from build123d import *

# Parameters (mm, degrees)
SKETCH_1_R               = 139
EXTRUDE_1_DEPTH          = 10
CUT_EXTRUDE_578_DEPTH    = 8
PATTERN_CIRCULAR_1_COUNT = 14
SKETCH_3_R               = 51
CUT_EXTRUDE_927_DEPTH    = 197.829875781
SKETCH_5_R               = 10
CUT_EXTRUDE_1077_DEPTH   = 197.738404995
PATTERN_CIRCULAR_2_COUNT = 14
HOLE_WIZARD_M3_D         = 3.6
MIRROR_2_COPY_1_D        = 3.6
M5SUPPORTINGPOLE_D       = 5.8
M5_SUPPORTING_POLE_D     = 5.8
MIRROR_4_COPY_1_D        = 5.8
MIRROR_4_COPY_2_D        = 5.8
MIRROR_4_COPY_3_D        = 5.8
SKETCH_15_R              = 5.1
CUT_EXTRUDE_7_DEPTH      = 5
MIRROR_6_COPY_1_SKETCH_R = 5.1
MIRROR_6_COPY_1_DEPTH    = 5
SKETCH_16_R              = 60
SKETCH_16_R_2            = 51
CUT_EXTRUDE_8_DEPTH      = 8
SKETCH_18_R              = 2.5
CUT_EXTRUDE_10_DEPTH     = 197.829875781


with BuildPart() as part:
    # ｽｹｯﾁ1 → ﾎﾞｽ - 押し出し1 (new body)
    with BuildSketch(Plane(origin=(0, 0, 0), x_dir=(1, 0, 0), z_dir=(0, 1, 0))):
        with Locations(Location((0, 0, 0), (0, 0, 270))):
            Circle(SKETCH_1_R)
    extrude(amount=EXTRUDE_1_DEPTH)

    # ｽｹｯﾁ2 → Cut-Extrude 578 (cut)
    with BuildSketch(Plane.XZ):
        with BuildLine():
            Line((18.5, 119), (18.5, 85))
            ThreePointArc((18.5, 85), (0, 66.5), (-18.5, 85))
            Line((-18.5, 85), (-18.5, 119))
            ThreePointArc((-18.5, 119), (0, 137.5), (18.5, 119))
        make_face()
    cut_extrude_578 = extrude(amount=-CUT_EXTRUDE_578_DEPTH, mode=Mode.SUBTRACT)

    # 円形ﾊﾟﾀｰﾝ1: Cut-Extrude 578 ×14 about axis
    pattern_circular_1_axis = Axis((0, 0, 0), (0, 1, 0))
    for i in range(1, PATTERN_CIRCULAR_1_COUNT):
        add(cut_extrude_578.rotate(pattern_circular_1_axis, i * 360 / PATTERN_CIRCULAR_1_COUNT), mode=Mode.SUBTRACT)

    # ｽｹｯﾁ3 → Cut-Extrude 927 (cut, through all)
    with BuildSketch(Plane(origin=(0, 0, 0), x_dir=(-1, 0, 0), z_dir=(0, -1, 0))):
        with Locations(Location((0, 0, 0), (0, 0, 90))):
            Circle(SKETCH_3_R)
    extrude(amount=-CUT_EXTRUDE_927_DEPTH, mode=Mode.SUBTRACT)

    # ｽｹｯﾁ5 → Cut-Extrude 1077 (cut, through all)
    with BuildSketch(Plane.XZ.offset(-8)):
        with Locations(Location((-6.5, 102, 0), (0, 0, 270))):
            Circle(SKETCH_5_R)
    cut_extrude_1077 = extrude(amount=-CUT_EXTRUDE_1077_DEPTH, mode=Mode.SUBTRACT)

    # 円形ﾊﾟﾀｰﾝ2: Cut-Extrude 1077 ×14 about axis
    pattern_circular_2_axis = Axis((0, 0, 0), (0, 1, 0))
    for i in range(1, PATTERN_CIRCULAR_2_COUNT):
        add(cut_extrude_1077.rotate(pattern_circular_2_axis, i * 360 / PATTERN_CIRCULAR_2_COUNT), mode=Mode.SUBTRACT)

    # M3(六角スペーサ) キールへの固定穴 (through all)
    with Locations(Plane(origin=(-31.622776602, 10, -45), x_dir=(0, 0, 1), z_dir=(0, 1, 0))):
        with Locations((0, 0)):
            hole_wizard_m3 = Hole(HOLE_WIZARD_M3_D / 2)

    # ﾐﾗｰ1: M3(六角スペーサ) キールへの固定穴 across plane
    add(hole_wizard_m3.mirror(Plane.XY), mode=Mode.SUBTRACT)

    # ﾐﾗｰ2: M3(六角スペーサ) キールへの固定穴 across plane
    add(hole_wizard_m3.mirror(Plane(origin=(0, 0, 0), x_dir=(0, 0, 1), z_dir=(1, 0, 0))), mode=Mode.SUBTRACT)

    # ﾐﾗｰ2 copy 1 (through all)
    with Locations(Plane(origin=(31.622776602, 10, 45), x_dir=(0, 0, -1), z_dir=(0, 1, 0))):
        with Locations((0, 0)):
            Hole(MIRROR_2_COPY_1_D / 2)

    # M5supportingpole用 (through all)
    with Locations(Plane(origin=(130, 0, 0), x_dir=(0, 0, -1), z_dir=(0, -1, 0))):
        with Locations((0, 0)):
            m5supportingpole = Hole(M5SUPPORTINGPOLE_D / 2)

    # M5 supporting_pole用 (through all)
    with Locations(Plane(origin=(81.053674242, 0, 101.638092721), x_dir=(0, 0, -1), z_dir=(0, -1, 0))):
        with Locations((0, 0)):
            m5_supporting_pole = Hole(M5_SUPPORTING_POLE_D / 2)

    # ﾐﾗｰ3: M5supportingpole用, M5 supporting_pole用 across plane
    add(m5supportingpole.mirror(Plane.XY), mode=Mode.SUBTRACT)
    add(m5_supporting_pole.mirror(Plane.XY), mode=Mode.SUBTRACT)

    # ﾐﾗｰ4: M5 supporting_pole用 across plane
    add(m5_supporting_pole.mirror(Plane(origin=(0, 0, 0), x_dir=(0, 0, 1), z_dir=(1, 0, 0))), mode=Mode.SUBTRACT)

    # ﾐﾗｰ4 copy 1 (through all)
    with Locations(Plane(origin=(-130, 0, 0), x_dir=(0, 0, 1), z_dir=(0, -1, 0))):
        with Locations((0, 0)):
            Hole(MIRROR_4_COPY_1_D / 2)

    # ﾐﾗｰ4 copy 2 (through all)
    with Locations(Plane(origin=(-81.053674242, 0, -101.638092721), x_dir=(0, 0, 1), z_dir=(0, -1, 0))):
        with Locations((0, 0)):
            Hole(MIRROR_4_COPY_2_D / 2)

    # ﾐﾗｰ4 copy 3 (through all)
    with Locations(Plane(origin=(-130, 0, 0), x_dir=(0, 0, -1), z_dir=(0, -1, 0))):
        with Locations((0, 0)):
            Hole(MIRROR_4_COPY_3_D / 2)

    # ｽｹｯﾁ15 → ｶｯﾄ - 押し出し7 (cut)
    with BuildSketch(Plane.XZ):
        with Locations(Location((81.053674242, 101.638092721, 0), (0, 0, 270))):
            Circle(SKETCH_15_R)
        with Locations(Location((130, 0, 0), (0, 0, 270))):
            Circle(SKETCH_15_R)
    cut_extrude_7 = extrude(amount=-CUT_EXTRUDE_7_DEPTH, mode=Mode.SUBTRACT)

    # ﾐﾗｰ5: ｶｯﾄ - 押し出し7 across plane
    add(cut_extrude_7.mirror(Plane.XY), mode=Mode.SUBTRACT)

    # ﾐﾗｰ6: ｶｯﾄ - 押し出し7 across plane
    add(cut_extrude_7.mirror(Plane(origin=(0, 0, 0), x_dir=(0, 0, 1), z_dir=(1, 0, 0))), mode=Mode.SUBTRACT)

    # ﾐﾗｰ6 copy 1 sketch → ﾐﾗｰ6 copy 1 (cut)
    with BuildSketch(Plane(origin=(0, 0, 0), x_dir=(-1, 0, 0), z_dir=(0, -1, 0))):
        with Locations(Location((81.053674242, 101.638092721, 0), (0, 0, 270))):
            Circle(MIRROR_6_COPY_1_SKETCH_R)
        with Locations(Location((130, 0, 0), (0, 0, 270))):
            Circle(MIRROR_6_COPY_1_SKETCH_R)
    extrude(amount=-MIRROR_6_COPY_1_DEPTH, mode=Mode.SUBTRACT)

    # ｽｹｯﾁ16 → ｶｯﾄ - 押し出し8 (cut)
    with BuildSketch(Plane.XZ):
        with Locations(Location((0, 0, 0), (0, 0, 270))):
            Circle(SKETCH_16_R)
        with Locations(Location((0, 0, 0), (0, 0, 270))):
            Circle(SKETCH_16_R_2, mode=Mode.SUBTRACT)
    extrude(amount=-CUT_EXTRUDE_8_DEPTH, mode=Mode.SUBTRACT)

    # ｽｹｯﾁ18 → ｶｯﾄ - 押し出し10 (cut, through all)
    with BuildSketch(Plane(origin=(0, 10, 0), x_dir=(1, 0, 0), z_dir=(0, 1, 0))):
        with Locations((139, 0)):
            Circle(SKETCH_18_R)
    extrude(amount=-CUT_EXTRUDE_10_DEPTH, mode=Mode.SUBTRACT)


solid = part.part
Read the model definition and answer for the solid it produces. Units are mm, in the model's axes. A direction names the side the tool comes from. Round coordinates to 2 decimals unless told otherwise and drop trailing zeros.
Q1. Each of these flat-tipped pins is pushed along its axis until it touches: pin 1 (12 mm diameter, centred on x = 91.5, z = -73, fed in from -Y); pin 2 (9.5 mm diameter, centred on x = -81.05, z = 101.64, fed in from -Y); pin 3 (5 mm diameter, centred on x = 43, y = 1, fed in from -Z). Where does it stop, or does it pass through?
Q2. Consider probe 1 along Z at (x, y) = (-62, 6.25); probe 2 along Z at (x, y) = (-92, 7.75); probe 3 along Z at (x, y) = (46.5, 3.25). Determine where each line is inside the solid, lowest interval first.
Q3. Which of the six approach directions +Z, -Z, +X, -X, +Y, -Y give full straight-line access (tool end or side, diameter ignored) to faces 1 (the face through (-6.06, 8.99, 111.99)), 2 (the face through (-81.278, 2.465, -106.733))?
Output:
1. pin 1: stops at y = 8
1. pin 2: stops at y = 5
1. pin 3: stops at z = -132.97
2. probe 1: z = -124.41 to -122.54, -86.11 to -73.11, -35.04 to 35.04, 73.11 to 86.11, 122.54 to 124.41
2. probe 2: z = -104.2 to -92.67, -49.71 to -39.97, -2.02 to 2.02, 39.97 to 49.71, 92.67 to 104.2
2. probe 3: z = -130.99 to -124.99, -60.78 to -37.92, 37.92 to 60.78, 124.99 to 130.99
3. face 1: +Y, -Y
3. face 2: -Y
